Can you work these out from the model? Positions are in its coordinate system, mm. Give positions to 0.01 mm unless a question says otherwise; leave off trailing zeros. Order: outer loops, then holes, each group sorted by start corner. A loop starts at its lowest first (then second) coordinate and runs counter-clockwise, first axis right, second up. Notation, with made-up numbers: M 87,-25 L 94,-25 A17 cw 94,-16 Z; hole C 87,-18.75 d7. An arc over 180 degrees is marked long. One line per question, with ' | ' between items. Start each with the question number.
1) If we section it at C-C, the plane x = -12.5: Please give me the cut outline in (y, z), plus the area to 3 significant figures.
2) If we section it at D-D, the plane z = -21.5: Please give me the cut outline in (x, y), plus the area to 3 significant figures.
3) I'm going to push flat-ended pins straight in: pin 1 Ø1.8 at (x, y) = (13.5, 11.5) entering from -Z; pin 2 Ø0.5 at (x, y) = (-13.5, 11) entering from -Z; pin 3 Ø0.5 at (y, z) = (11, 5.5) entering from +X. Where does each tip first touch, or does it pass through?
4) Please list where these lines run through material, in increasing order: line 1 along Z through (x, y) = (0, 10.95); line 2 along Z through (x, y) = (0, 10.15); line 3 along Z through (x, y) = (16, 9.5). Write a range as [from, to].
5) If we section it at B-B, the plane z = -6: Please give me the cut outline in (x, y).
6) If we section it at A-A, the plane y = 2.5: Please give me the cut outline in (x, z).
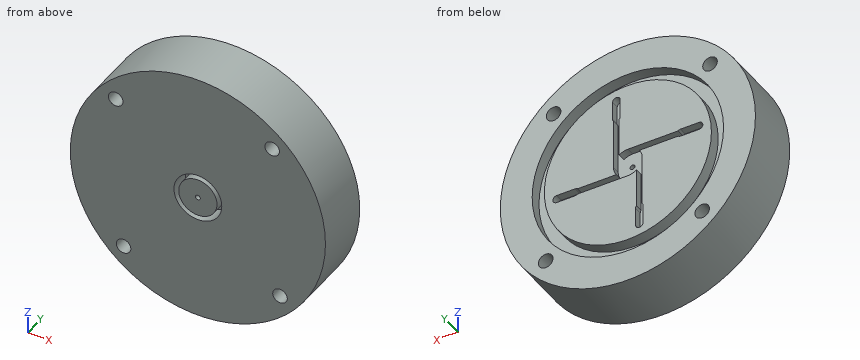
Autodesk Inventor part; units mm, degrees
ref_plane "YZ Plane" through (0, 0, 0) normal (1, 0, 0) x (0, 1, 0)
ref_plane "XZ Plane" through (0, 0, 0) normal (0, 1, 0) x (-1, 0, 0)
ref_plane "XY Plane" through (0, 0, 0) normal (0, 0, 1) x (1, 0, 0)
sketch "Sketch1" plane through (0, 0, 0) normal (0, 1, 0) x (-1, 0, 0)
  circle A0 centre (0, 0) radius 0.508
  circle A1 centre (0, 0) radius 3
  line L0 (1.8062, -2.3953) -> (1.8062, -10.5053)
  arc A2 (1.6092, -14.8779) -> (3.197, -14.8779) centre (2.4031, -14.8779) ccw
  line L1 (3.197, -14.8779) -> (3.197, -11.0287)
  line L2 (1.6092, -14.8779) -> (1.6092, -11.0287)
  line L3 (3, 0) -> (3, -10.5053)
  arc A3 (3.197, -11.0287) -> (3, -10.5053) centre (2.4031, -11.0287) ccw
  arc A4 (1.8062, -10.5053) -> (1.6092, -11.0287) centre (2.4031, -11.0287) ccw
  line L4 (0, 3) -> (10.5053, 3)
  line L5 (14.8779, 3.197) -> (11.0287, 3.197)
  line L6 (14.8779, 1.6092) -> (11.0287, 1.6092)
  arc A5 (14.8779, 1.6092) -> (14.8779, 3.197) centre (14.8779, 2.4031) ccw
  arc A6 (11.0287, 3.197) -> (10.5053, 3) centre (11.0287, 2.4031) ccw
  arc A7 (10.5053, 1.8062) -> (11.0287, 1.6092) centre (11.0287, 2.4031) ccw
  line L7 (2.3953, 1.8062) -> (10.5053, 1.8062)
  line L8 (-3, 0) -> (-3, 10.5053)
  line L9 (-3.197, 14.8779) -> (-3.197, 11.0287)
  line L10 (-1.6092, 14.8779) -> (-1.6092, 11.0287)
  arc A8 (-1.6092, 14.8779) -> (-3.197, 14.8779) centre (-2.4031, 14.8779) ccw
  arc A9 (-3.197, 11.0287) -> (-3, 10.5053) centre (-2.4031, 11.0287) ccw
  arc A10 (-1.8062, 10.5053) -> (-1.6092, 11.0287) centre (-2.4031, 11.0287) ccw
  line L11 (-1.8062, 2.3953) -> (-1.8062, 10.5053)
  line L12 (0, -3) -> (-10.5053, -3)
  line L13 (-14.8779, -3.197) -> (-11.0287, -3.197)
  line L14 (-14.8779, -1.6092) -> (-11.0287, -1.6092)
  arc A11 (-14.8779, -1.6092) -> (-14.8779, -3.197) centre (-14.8779, -2.4031) ccw
  arc A12 (-11.0287, -3.197) -> (-10.5053, -3) centre (-11.0287, -2.4031) ccw
  arc A13 (-10.5053, -1.8062) -> (-11.0287, -1.6092) centre (-11.0287, -2.4031) ccw
  line L15 (-2.3953, -1.8062) -> (-10.5053, -1.8062)
  circle A14 centre (0, 0) radius 17.4625
  circle A15 centre (0, 0) radius 20.0025
  circle A16 centre (0, 0) radius 26.67
  line L16 (0, 0) -> (26.67, 0) construction
  circle A17 centre (15.5308, -17.1702) radius 1.524
  circle A18 centre (17.1702, 15.5308) radius 1.524
  circle A19 centre (-15.5308, 17.1702) radius 1.524
  circle A20 centre (-17.1702, -15.5308) radius 1.524
  arc A21 (3.197, -11.0287) -> (1.6092, -11.0287) centre (2.4031, -11.0287) ccw
  arc A22 (11.0287, 3.197) -> (11.0287, 1.6092) centre (11.0287, 2.4031) ccw
  arc A23 (-3.197, 11.0287) -> (-1.6092, 11.0287) centre (-2.4031, 11.0287) ccw
  arc A24 (-11.0287, -3.197) -> (-11.0287, -1.6092) centre (-11.0287, -2.4031) ccw
  line L17 (0, 0) -> (14.8779, 0)
  line L18 (17.0946, 3.5656) -> (17.0946, 3)
  line L19 (17.0946, 1.8062) -> (17.0946, 1.6092)
  point P0 (2.4031, -15.6718)
  dimension "d16" = 34.925
  dimension "d0" = 1.016
  dimension "d1" = 6
  dimension "d13" = 360
  dimension "d17" = 40.005
  dimension "d18" = 53.34
  dimension "d24" = 360
  dimension "d28" = 360
  dimension "d44" = 17.1702
extrude "Extrusion1" add sketch "Sketch1" along normal blind 12 contours A14 | A16
extrude "Extrusion2" add sketch "Sketch1" along normal blind 10.3632 contours A1 | L3 A21 L0 A1 | A1 L4 A22 L7 | A3 L1 A2 L2 A4 A21 | A22 A6 L5 A5 L6 A7 | L12 A24 L15 A1 | A1 L8 A23 L11 | A12 L13 A11 L14 A13 A24 | A23 A9 L9 A8 L10 A10
extrude "Extrusion3" add sketch "Sketch1" along normal blind 9.6215 contours A15
thread "Thread1"
thread "Thread2"
thread "Thread3"
thread "Thread4"
sketch "Sketch2" plane through (0, 0, 0) normal (0, -1, 0) x (1, 0, 0)
  circle A0 centre (0, 0) radius 4
  circle A1 centre (0, 0) radius 0.508
  circle A2 centre (0, 0) radius 5
  dimension "d46" = 8
  dimension "d47" = 10
extrude "Extrusion4" cut sketch "Sketch2" against normal blind 4 contours A2
thread "Thread5"
Results found:
1) outline: M 0,-23.56 L 12,-23.56 L 12,-15.62 L 9.62,-15.62 L 9.62,-12.19 L 12,-12.19 L 12,1.61 L 10.36,1.61 L 10.36,3.2 L 12,3.2 L 12,12.19 L 9.62,12.19 L 9.62,15.62 L 12,15.62 L 12,23.56 L 0,23.56 Z | area: 547 mm²
2) outline: M -15.78,0 L 15.78,0 L 15.78,12 L -15.78,12 Z | area: 379 mm²
3) pin 1: stops at z = -23.51 | pin 2: stops at z = -23.15 | pin 3: stops at x = 26.15
4) line 1: z = [-26.67, -20], [-17.46, -3], [3, 17.46], [20, 26.67] | line 2: z = [-26.67, -20], [-17.46, -0.51], [0.51, 17.46], [20, 26.67] | line 3: z = [-21.34, -16.51], [-14.55, 15.72], [18.62, 21.34]
5) outline: M -25.99,0 L 25.99,0 L 25.99,12 L 19.08,12 L 19.08,9.62 L 16.4,9.62 L 16.4,12 L -1.81,12 L -1.81,10.36 L -3,10.36 L -3,12 L -16.4,12 L -16.4,9.62 L -19.08,9.62 L -19.08,12 L -25.99,12 Z
6) outline: C 0,0 d53.34; C 0,0 d8; hole C -17.17,15.53 d3.05; hole C -15.53,-17.17 d3.05; hole C 0,0 d10; hole C 0,0 d1.02; hole C 15.53,17.17 d3.05; hole C 17.17,-15.53 d3.05
